from build123d import *

# Parameters (mm, degrees)
SKETCH_1_W                  = 79
SKETCH_1_H                  = 160
EXTRUDE_300_DEPTH           = 10
HOLE_WIZARD_M3_D            = 3.4
HOLE_WIZARD_M3_CSINK_D      = 6.3
HOLE_WIZARD_M3_CSINK_ANGLE  = 90
HOLE_WIZARD_M6_D            = 6.6
HOLE_WIZARD_M6_CSINK_D      = 12.6
HOLE_WIZARD_M6_CSINK_ANGLE  = 90
HOLE_WIZARD_M61_D           = 5
HOLE_WIZARD_M61_DEPTH       = 35
HOLE_WIZARD_M61_CSINK_D     = 6.05
HOLE_WIZARD_M61_CSINK_ANGLE = 90
HOLE_WIZARD_M61_TIP         = 1.502151548


with BuildPart() as part:
    # Эскиз1 → Extrude 300 (new body)
    with BuildSketch(Plane(origin=(0, 0, 0), x_dir=(1, 0, 0), z_dir=(0, 1, 0))):
        Rectangle(SKETCH_1_W, SKETCH_1_H)
    extrude(amount=EXTRUDE_300_DEPTH)

    # Каретки M3 (through all)
    with Locations(Plane(origin=(0, 10, 0), x_dir=(1, 0, 0), z_dir=(0, 1, 0))):
        with Locations((9, -56.5), (34, -56.5), (34, -31.5), (9, -31.5), (9, 56.5), (9, 31.5), (34, 31.5), (34, 56.5)):
            CounterSinkHole(HOLE_WIZARD_M3_D / 2, HOLE_WIZARD_M3_CSINK_D / 2, counter_sink_angle=HOLE_WIZARD_M3_CSINK_ANGLE)

    # КреплениеПлиты-M6 (through all)
    with Locations(Plane(origin=(0, 10, 0), x_dir=(1, 0, 0), z_dir=(0, 1, 0))):
        with Locations((-18.5, 25), (-18.5, -25)):
            CounterSinkHole(HOLE_WIZARD_M6_D / 2, HOLE_WIZARD_M6_CSINK_D / 2, counter_sink_angle=HOLE_WIZARD_M6_CSINK_ANGLE)

    # Отверстие обработанное метчиком M61
    with Locations(Plane.ZY.offset(39.5)):
        with Locations((-40, 5), (40, 5)):
            CounterSinkHole(HOLE_WIZARD_M61_D / 2, HOLE_WIZARD_M61_CSINK_D / 2, depth=HOLE_WIZARD_M61_DEPTH, counter_sink_angle=HOLE_WIZARD_M61_CSINK_ANGLE)
            with Locations((0, 0, -(HOLE_WIZARD_M61_DEPTH + HOLE_WIZARD_M61_TIP / 2))):  # 118° drill point
                Cone(0, HOLE_WIZARD_M61_D / 2, HOLE_WIZARD_M61_TIP, mode=Mode.SUBTRACT)


solid = part.part
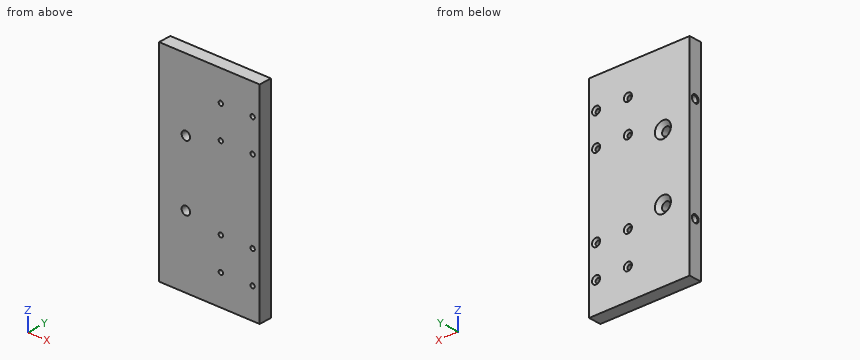
Geometry check sheet. Reference: the model listing, model coordinates, mm. Coordinates: 2 decimals unless noted, no trailing zeros. Loops run counter-clockwise (first coordinate to the right, second up) from the corner with the lowest first, then second, coordinate; pieces in that order, holes last. Notation, with made-up numbers: (-26, -36.75) - (-5, -36.75) arc R15 cw to (-5, -27.75) - close; hole circle Ø10 at (61, -32). An arc over 180 degrees is marked (long way). Use one line per item in the form item = value. Start each with the question number.
Item 1: Section check B-B, the plane x = 34. Enter the section's corners in (y, z).
Item 2: Section check A-A, the plane z = 25. Enter the section's corners in (x, y).
Item 3: Section check D-D, the plane x = -17. Give the number of separate pieces and of enclosed holes in the cut face, and give its area (3 significant figures).
Item 4: Gauge pin test, flat ends, axial feed: pin 1 (1 mm diameter, centred on x = 11, z = -12.5, fed in from -Y); pin 2 (4 mm diameter, centred on y = 5, z = -40, fed in from -X); pin 3 (10.5 mm diameter, centred on x = -18.5, z = -25, fed in from +Y); pin 4 (5.5 mm diameter, centred on x = 34, z = 56.5, fed in from +Y). Record the tip position at first contact, or that the pin passes through.
Item 5: Section check C-C, the plane z = 56.5. Enter the section's corners in (x, y).
Item 6: Thickness scan on probe 1 along X at (y, z) = (3.25, -56.5); probe 2 along Z at (x, y) = (9, 4); probe 3 along Z at (x, y) = (-16, 5.75). Record the ranges inside material, lowest first.
Computed:
q1.outline = (0, -80) - (10, -80) - (10, -59.65) - (8.55, -58.2) - (0, -58.2) - close; (0, -54.8) - (8.55, -54.8) - (10, -53.35) - (10, -34.65) - (8.55, -33.2) - (0, -33.2) - close; (0, -29.8) - (8.55, -29.8) - (10, -28.35) - (10, 28.35) - (8.55, 29.8) - (0, 29.8) - close; (0, 33.2) - (8.55, 33.2) - (10, 34.65) - (10, 53.35) - (8.55, 54.8) - (0, 54.8) - close; (0, 58.2) - (8.55, 58.2) - (10, 59.65) - (10, 80) - (0, 80) - close
q2.outline = (-39.5, 0) - (-21.8, 0) - (-21.8, 7) - (-24.8, 10) - (-39.5, 10) - close; (-15.2, 0) - (39.5, 0) - (39.5, 10) - (-12.2, 10) - (-15.2, 7) - close
q3.separate_pieces = 3
q3.enclosed_holes = 2
q3.area = 1,420 mm2
q4.pin_1 = 0
q4.pin_2 = -4.2
q4.pin_3 = 8.95
q4.pin_4 = 9.6
q5.outline = (-39.5, 0) - (7.3, 0) - (7.3, 8.55) - (5.85, 10) - (-39.5, 10) - close; (10.7, 0) - (32.3, 0) - (32.3, 8.55) - (30.85, 10) - (12.15, 10) - (10.7, 8.55) - close; (35.7, 0) - (39.5, 0) - (39.5, 10) - (37.15, 10) - (35.7, 8.55) - close
q6.probe_1 = -39.5 to 7.3, 10.7 to 32.3, 35.7 to 39.5
q6.probe_2 = -80 to -58.2, -54.8 to -33.2, -29.8 to 29.8, 33.2 to 54.8, 58.2 to 80
q6.probe_3 = -80 to -42.38, -37.62 to -27.15, -22.85 to 22.85, 27.15 to 37.62, 42.38 to 80
